Here's how the part is built. I have some questions about the finished solid (model axes, mm). A direction names the side the tool comes from. Coordinates: 2 decimals unless noted, no trailing zeros. Order: outer loops, then holes, each group sorted by start corner. A loop starts at its lowest first (then second) coordinate and runs counter-clockwise, first axis right, second up.
```python
from build123d import *

# Parameters (mm, degrees)
SKETCH1_W           = 7.55
SKETCH1_H           = 5.75
BOSS_EXTRUDE1_DEPTH = 3
FILLET1_R           = 2.5
CUT_EXTRUDE1_DEPTH  = 3


with BuildPart() as part:
    # Sketch1 → Boss-Extrude1 (new body)
    with BuildSketch(Plane.XY):
        with BuildLine():
            Line((-8.11, 12.5), (-8.11, -12.5))
            ThreePointArc((-8.11, -12.5), (0, -20.61), (8.11, -12.5))
            Line((8.11, -12.5), (8.11, 12.5))
            ThreePointArc((8.11, 12.5), (0, 20.61), (-8.11, 12.5))
        make_face()
        with Locations((0, 12.5)):
            Rectangle(SKETCH1_W, SKETCH1_H, mode=Mode.SUBTRACT)
    extrude(amount=BOSS_EXTRUDE1_DEPTH)

    # Fillet1
    fillet1_edges = [part.edges().sort_by_distance(p)[0] for p in [
        (3.775, 9.625, 1.5),
        (3.775, 15.375, 1.5),
        (-3.775, 15.375, 1.5),
        (-3.775, 9.625, 1.5),
    ]]
    fillet(fillet1_edges, radius=FILLET1_R)

    # Sketch2 → Cut-Extrude1 (cut)
    with BuildSketch(Plane.XY.offset(3)):
        with BuildLine():
            Line((-2.75, -9.75), (-2.75, -15.25))
            ThreePointArc((-2.75, -15.25), (0, -16.389087297), (2.75, -15.25))
            Line((2.75, -15.25), (2.75, -9.75))
            ThreePointArc((2.75, -9.75), (0, -8.610912703), (-2.75, -9.75))
        make_face()
    extrude(amount=-CUT_EXTRUDE1_DEPTH, mode=Mode.SUBTRACT)


solid = part.part
```
Q1. If we section it at A-A on x = 0: Write out the boundary of the cut face in (y, z) (3 decimals), then the cut area to 3 significant figures.
Q2. If we section it at B-B on z = 1.7: Write out the boundary of the cut face in (x, y) (3 decimals).
Q3. If we section it at D-D on y = -16: Write out the boundary of the cut face in (x, z).
Q4. We'd pull the mould along Y, two halves only. Please class faces 1 (the cylindrical face through (-0.18, -20.61, 1.48)), 2 (the flat face through (8.11, 0, 1)), 3 (the cylindrical face through (0.04, -8.61, 1.52)): pulls with the +Y half, pulls with the -Y half, needs draft (parallel to the pull), parting line crosses it, or undercut.
Q5. Will these pins go through, and if not, where does the flat tip stop? pin 1 (1 mm diameter, centred on x = 1, z = 2.5, fed in from -Y); pin 2 (8 mm diameter, centred on x = -2.5, y = -10.5, fed in from +Z).
Q6. For faces 4 (the cylindrical face through (-3.023, 10.338, 1.521)), 5 (the flat face through (0, 0, 0)), which set-ups out of +Z, -Z, +X, -X, +Y, -Y let a thin tool reach every point of the face, with its end or its side?
Q7. I need wall thicknesses on L1, parallel to Y at x = 0, z = 0.65 (3 decimals); L2, parallel to Y at x = -2.5, z = 0.4; L3, parallel to X at y = -9.5, z = 0.55. Which ranges of each line are inside material? Lowest first, please.
Q8. If we section it at C-C on y = -11: Write out the boundary of the cut face in (x, z), then the cut area to 3 significant figures.
Reply:
1. outline: (-20.61, 0) - (-16.389, 0) - (-16.389, 3) - (-20.61, 3) - close; (-8.611, 0) - (9.625, 0) - (9.625, 3) - (-8.611, 3) - close; (15.375, 0) - (20.61, 0) - (20.61, 3) - (15.375, 3) - close
1. area: 83.1 mm2
2. outline: (-8.11, -12.5) arc R8.11 ccw to (8.11, -12.5) - (8.11, 12.5) arc R8.11 ccw to (-8.11, 12.5) - close; hole (-3.775, 12.125) arc R2.5 ccw to (-1.275, 9.625) - (1.275, 9.625) arc R2.5 ccw to (3.775, 12.125) - (3.775, 12.875) arc R2.5 ccw to (1.275, 15.375) - (-1.275, 15.375) arc R2.5 ccw to (-3.775, 12.875) - close; hole (-2.75, -15.25) arc R3.889 ccw to (2.75, -15.25) - (2.75, -9.75) arc R3.889 ccw to (-2.75, -9.75) - close
3. outline: (-7.32, 0) - (-1.7, 0) - (-1.7, 3) - (-7.32, 3) - close; (1.7, 0) - (7.32, 0) - (7.32, 3) - (1.7, 3) - close
4. face 1: pulls with the -Y half
4. face 2: needs draft
4. face 3: undercut
5. pin 1: stops at y = -20.59
5. pin 2: stops at z = 3
6. face 4: +Z, -Z
6. face 5: -Z, +X, -X, +Y, -Y
7. L1: y = -20.61 to -16.389, -8.611 to 9.625, 15.375 to 20.61
7. L2: y = -20.22 to -15.48, -9.52 to 9.95, 15.05 to 20.22
7. L3: x = -8.11 to -2.47, 2.47 to 8.11
8. outline: (-8.11, 0) - (-2.75, 0) - (-2.75, 3) - (-8.11, 3) - close; (2.75, 0) - (8.11, 0) - (8.11, 3) - (2.75, 3) - close
8. area: 32.2 mm2
